Could you check a few things on this model? Use its own coordinates, in mm. A direction names the side the tool comes from. Give positions to 0.01 mm unless a question says otherwise; leave off trailing zeros. Write each loop counter-clockwise with the first axis right and the second up, starting at its lowest first coordinate (ties: lowest second). Pieces come first, ordered by that corner, then holes. Notation, with made-up numbers: (61, -29.75) - (102, -29.75) arc R15 ccw to (102, -18.75) - close; hole circle Ø4 at (-13, 19.25). An arc over 180 degrees is marked (long way). Answer in a Markdown table with one row per item.
from build123d import *

# Parameters (mm, degrees)
SCHIZZO9_W                     = 45.3
SCHIZZO9_H                     = 22
BASE_FLANGIA2_DEPTH            = 2
BORDO_FLANGIA2_STRIP_W         = 9.4732
BORDO_FLANGIA2_STRIP_H         = 2
BORDO_FLANGIA2_STRIP_CUT_DEPTH = 45.3
BORDO_FLANGIA2_DEPTH           = 45.3
BORDO_FLANGIA3_STRIP_W         = 9.4732
BORDO_FLANGIA3_STRIP_H         = 2
BORDO_FLANGIA3_STRIP_CUT_DEPTH = 45.3
BORDO_FLANGIA3_DEPTH           = 45.3
SCHIZZO22_R                    = 11
TAGLIO_ESTRUSIONE1_DEPTH       = 10


# Sheet-metal steps are written as plain solids
with BuildPart() as part:
    # Schizzo9 → Base-Flangia2 (new body)
    with BuildSketch(Plane(origin=(0, 0, 0), x_dir=(0, 0, -1), z_dir=(1, 0, 0))):
        with Locations((22.65, -11)):
            Rectangle(SCHIZZO9_W, SCHIZZO9_H)
    extrude(amount=-BASE_FLANGIA2_DEPTH)

    # Bordo-Flangia2 strip (across the edge) → Bordo-Flangia2 strip cut (cut)
    with BuildSketch(Plane(origin=(0, 0, -45.3), x_dir=(0, -1, 0), z_dir=(0, 0, 1))):
        with Locations((-2, -1)):
            Rectangle(BORDO_FLANGIA2_STRIP_W, BORDO_FLANGIA2_STRIP_H)
    extrude(amount=BORDO_FLANGIA2_STRIP_CUT_DEPTH, mode=Mode.SUBTRACT)

    # Bordo-Flangia2 section (across the edge) → Bordo-Flangia2 (add)
    with BuildSketch(Plane(origin=(0, 0, -45.3), x_dir=(0, -1, 0), z_dir=(0, 0, 1))):
        with BuildLine():
            Line((0, 0.7366), (0, 47.143791264))
            Line((0, 47.143791264), (2, 47.143791264))
            Line((2, 47.143791264), (2, 0.7366))
            ThreePointArc((2, 0.7366), (2.215745145, 0.215745145), (2.7366, 0))
            Line((2.7366, 0), (2.7366, -2))
            ThreePointArc((2.7366, -2), (0.801531583, -1.198468417), (0, 0.7366))
        make_face()
    extrude(amount=BORDO_FLANGIA2_DEPTH)

    # Bordo-Flangia3 strip (across the edge) → Bordo-Flangia3 strip cut (cut)
    with BuildSketch(Plane(origin=(47.143791264, 0, 0), x_dir=(-1, 0, 0), z_dir=(0, 0, -1))):
        with Locations((-2, -1)):
            Rectangle(BORDO_FLANGIA3_STRIP_W, BORDO_FLANGIA3_STRIP_H)
    extrude(amount=BORDO_FLANGIA3_STRIP_CUT_DEPTH, mode=Mode.SUBTRACT)

    # Bordo-Flangia3 section (across the edge) → Bordo-Flangia3 (add)
    with BuildSketch(Plane(origin=(47.143791264, 0, 0), x_dir=(-1, 0, 0), z_dir=(0, 0, -1))):
        with BuildLine():
            Line((0, 0.7366), (0, 43))
            Line((0, 43), (2, 43))
            Line((2, 43), (2, 0.7366))
            ThreePointArc((2, 0.7366), (2.215745145, 0.215745145), (2.7366, 0))
            Line((2.7366, 0), (2.7366, -2))
            ThreePointArc((2.7366, -2), (0.801531583, -1.198468417), (0, 0.7366))
        make_face()
    extrude(amount=BORDO_FLANGIA3_DEPTH)

    # Schizzo22 → Taglio-Estrusione1 (cut)
    with BuildSketch(Plane(origin=(47.143791264, 0, 0), x_dir=(0, 0, -1), z_dir=(1, 0, 0))):
        with Locations((22.65, 21.8683)):
            Circle(SCHIZZO22_R)
    extrude(amount=-TAGLIO_ESTRUSIONE1_DEPTH, mode=Mode.SUBTRACT)


solid = part.part
1) On a 3-axis mill with a long thin cutter (end or side, diameter ignored), from which of +Z, -Z, +X, -X, +Y, -Y can I reach the whole of each face in a straight line? I mean faces 4 (the face through (-2, -12, -22)), 5 (the face through (22, 0, -23)), 6 (the face through (23, -2, -23)). Say none if no direction works.
Check values:
| item | result |
|---|---|
| face 4 | +Z, -Z, -X, +Y, -Y |
| face 5 | +Z, -Z, -X, +Y |
| face 6 | +Z, -Z, +X, -Y |
2) We'd pull the mould along Z, two halves only. Please class faces 1 (the face through (46.16, 22.35, -11.66)), 2 (the face through (0, -12, -22)), 3 (the face through (26, -1, -45.3)): +Z half, -Z half, draft (parallel to the pull), parting line (faces both ways), or undercut.
Check values:
| item | result |
|---|---|
| face 1 | undercut |
| face 2 | draft |
| face 3 | -Z half |
3) Imagine slicing it at A-A (z = -22.65). List the corners of the cut face in (x, y) for me, then the cut area to 3 significant figures.
Check values:
| item | result |
|---|---|
| outline | (-2, -22) - (0, -22) - (0, -2.74) arc R0.74 cw to (0.74, -2) - (44.41, -2) arc R2.74 ccw to (47.14, 0.74) - (47.14, 10.87) - (45.14, 10.87) - (45.14, 0.74) arc R0.74 cw to (44.41, 0) - (0.74, 0) arc R2.74 ccw to (-2, -2.74) - close; (45.14, 32.87) - (47.14, 32.87) - (47.14, 43) - (45.14, 43) - close |
| area | 177 mm2 |
4) Imagine slicing it at D-D (y = -4.5). List the corners of the cut face in (x, z) for me, then the cut area to 3 significant figures.
Check values:
| item | result |
|---|---|
| outline | (-2, -45.3) - (0, -45.3) - (0, 0) - (-2, 0) - close |
| area | 90.6 mm2 |
5) If I drill on line 1 (X direction, y = 20, z = -37); line 2 (X direction, y = -18.5, z = -20), over which ranges is the centre line in solid material (lowest first)?
Check values:
| item | result |
|---|---|
| line 1 | x = 45.14 to 47.14 |
| line 2 | x = -2 to 0 |
6) Imagine slicing it at C-C (z = -35). List the corners of the cut face in (x, y) for me, then the cut area to 3 significant figures.
Check values:
| item | result |
|---|---|
| outline | (-2, -22) - (0, -22) - (0, -2.74) arc R0.74 cw to (0.74, -2) - (44.41, -2) arc R2.74 ccw to (47.14, 0.74) - (47.14, 43) - (45.14, 43) - (45.14, 0.74) arc R0.74 cw to (44.41, 0) - (0.74, 0) arc R2.74 ccw to (-2, -2.74) - close |
| area | 221 mm2 |
7) Will these pins go through, and if not, where does the flat tip stop? P1, Ø5, axis at x = 25.5, z = -7, coming from the +Y side; P2, Ø15.5, axis at y = -9, z = -15, coming from the +X side; P3, Ø8, axis at x = 41, z = -14.5, coming from the -Y side.
Check values:
| item | result |
|---|---|
| P1 | stops at y = 0 |
| P2 | stops at x = 46.29 |
| P3 | stops at y = -2 |
8) Imagine slicing it at B-B (y = 27). List the corners of the cut face in (x, z) for me.
Check values:
| item | result |
|---|---|
| outline | (45.14, -45.3) - (47.14, -45.3) - (47.14, -32.38) - (45.14, -32.38) - close; (45.14, -12.92) - (47.14, -12.92) - (47.14, 0) - (45.14, 0) - close |
